```python
from build123d import *

# Parameters (mm, degrees)
SKETCH1_R               = 1.6
SKETCH1_R_2             = 1.15
SKETCH1_R_3             = 1.33
BASE_SHAPE_DEPTH        = 1.75
MILLING_FILLETS_R       = 1
SKETCH3_R               = 3
SCREW_HEAD_CUT_DEPTH    = 0.3
SCREW_HEAD_CHAMFER_SIZE = 1.4


with BuildPart() as part:
    # Sketch1 → Base shape (new body)
    with BuildSketch(Plane(origin=(0, 0, 0), x_dir=(1, 0, 0), z_dir=(0, 1, 0))):
        with BuildLine():
            Line((15.5, 39.2), (-15.5, 39.2))
            ThreePointArc((-15.5, 39.2), (-18.328427125, 38.028427125), (-19.5, 35.2))
            Line((-19.5, 35.2), (-19.5, -19.5))
            Line((-19.5, -19.5), (19.5, -19.5))
            Line((19.5, -19.5), (19.5, 35.2))
            ThreePointArc((19.5, 35.2), (18.328427125, 38.028427125), (15.5, 39.2))
        make_face()
        with Locations(Location((-15.25, -15.25, 0), (0, 0, 270))):
            Circle(SKETCH1_R, mode=Mode.SUBTRACT)
        with Locations(Location((15.25, -15.25, 0), (0, 0, 270))):
            Circle(SKETCH1_R, mode=Mode.SUBTRACT)
        with BuildLine():
            ThreePointArc((-17.7, 13.606832327), (-13.284874461, 13.049822367), (-13.341630288, 17.499583304))
            Line((-13.341630288, 17.499583304), (7.05, 17.499583304))
            Line((7.05, 17.499583304), (7.05, 17.05))
            ThreePointArc((7.05, 17.05), (8.336587223, 15.08098543), (10.656528722, 15.46853736))
            ThreePointArc((10.656528722, 15.46853736), (11.674639953, 15.673161101), (12.325380263, 14.863866097))
            ThreePointArc((12.325380263, 14.863866097), (14.578174541, 12.377518398), (17.7, 13.606832327))
            Line((17.7, 13.606832327), (17.7, -13.606832327))
            ThreePointArc((17.7, -13.606832327), (13.284874461, -13.049822367), (13.341630288, -17.499583304))
            Line((13.341630288, -17.499583304), (-13.341630288, -17.499583304))
            ThreePointArc((-13.341630288, -17.499583304), (-13.284874461, -13.049822367), (-17.7, -13.606832327))
            Line((-17.7, -13.606832327), (-17.7, 13.606832327))
        make_face(mode=Mode.SUBTRACT)
        with Locations(Location((-15.25, 15.25, 0), (0, 0, 270))):
            Circle(SKETCH1_R, mode=Mode.SUBTRACT)
        with Locations(Location((-15.25, 33.25, 0), (0, 0, 270))):
            Circle(SKETCH1_R, mode=Mode.SUBTRACT)
        with Locations(Location((9.2, 17.05, 0), (0, 0, 270))):
            Circle(SKETCH1_R_2, mode=Mode.SUBTRACT)
        with Locations(Location((15.25, 15.25, 0), (0, 0, 270))):
            Circle(SKETCH1_R, mode=Mode.SUBTRACT)
        with Locations(Location((3.5, 26.95, 0), (0, 0, 270))):
            Circle(SKETCH1_R_3, mode=Mode.SUBTRACT)
        with Locations(Location((15.25, 33.25, 0), (0, 0, 270))):
            Circle(SKETCH1_R, mode=Mode.SUBTRACT)
    extrude(amount=BASE_SHAPE_DEPTH)

    # Milling fillets
    milling_fillets_edges = [part.edges().sort_by_distance(p)[0] for p in [
        (-17.7, 0.875, 13.606832327),
        (-13.341630288, 0.875, 17.499583304),
        (13.341630288, 0.875, 17.499583304),
        (17.7, 0.875, 13.606832327),
        (17.7, 0.875, -13.606832327),
        (-13.341630288, 0.875, -17.499583304),
        (-17.7, 0.875, -13.606832327),
        (7.05, 0.875, -17.499583304),
    ]]
    fillet(milling_fillets_edges, radius=MILLING_FILLETS_R)

    # Sketch3 → Screw head cut (cut)
    with BuildSketch(Plane(origin=(0, 1.75, 0), x_dir=(1, 0, 0), z_dir=(0, 1, 0))):
        with Locations(Location((-15.25, 33.25, 0), (0, 0, 270))):
            Circle(SKETCH3_R)
        with Locations(Location((15.25, 33.25, 0), (0, 0, 270))):
            Circle(SKETCH3_R)
    extrude(amount=-SCREW_HEAD_CUT_DEPTH, mode=Mode.SUBTRACT)

    # Screw head chamfer
    screw_head_chamfer_edges = [part.edges().sort_by_distance(p)[0] for p in [
        (-15.25, 1.45, -34.85),
        (15.25, 1.45, -34.85),
    ]]
    chamfer(screw_head_chamfer_edges, length=SCREW_HEAD_CHAMFER_SIZE - 0.0001)  # a hair under: the kernel refuses the full size


solid = part.part
```
CAD build for the part. Positions are in the model's coordinates, mm. A direction names the side the tool comes from. Round coordinates to 2 decimals unless told otherwise and drop trailing zeros. Order: outer loops, then holes, each group sorted by start corner. A loop starts at its lowest first (then second) coordinate and runs counter-clockwise, first axis right, second up.
Item 1: Saw through at A-A on x = -1. Write the cut outline in (y, z), then the cut area to 3 significant figures.
Item 2: Saw through at C-C on z = -33.25. State how many separate pieces and enclosed holes the cut face has, then the cut area to 3 significant figures.
Item 3: Probe line 1 along X through (y, z) = (0.05, -33.25); line 2 along X through (y, z) = (1.55, -33.25); line 3 along X through (y, z) = (0.85, 15.25). List the from-to ranges inside material, lowest first.
Item 4: Saw through at B-B on z = -26.95. Write the cut outline in (x, y), then the cut area to 3 significant figures.
Item 5: Tool access for faces 5 (the face through (-12.322, 0.887, -17.073)), 6 (the face through (0, 1, -39.2)): list every direction of +Z, -Z, +X, -X, +Y, -Y with a clear straight run to the whole face (end or side of a thin tool).
Item 6: Mould opens along Z. For faces 1 (the face through (-12.322, 0.887, 17.073)), 2 (the face through (-18.297, 0.863, -38.059)), 3 (the face through (3.9, 0.86, -25.68)), 4 (the face through (-19.5, 1, -8)) say: pulls with the +Z half, pulls with the -Z half, needs draft (parallel to the pull), parting line crosses it, or undercut.
Item 7: Pin check, flat tips, straight feed: pin 1 (1.4 mm diameter, centred on x = 9.2, z = -17.05, fed in from +Y); pin 2 (1.8 mm diameter, centred on x = -16, z = -33.5, fed in from +Y); pin 3 (5 mm diameter, centred on x = 15.25, z = -33.25, fed in from +Y). Stop position of each tip, or through.
Reported:
1. outline: (0, -39.2) - (1.75, -39.2) - (1.75, -17.5) - (0, -17.5) - close; (0, 17.5) - (1.75, 17.5) - (1.75, 19.5) - (0, 19.5) - close
1. area: 41.5 mm2
2. separate pieces: 3
2. enclosed holes: 0
2. area: 51.5 mm2
3. line 1: x = -19.5 to -16.85, -13.65 to 13.65, 16.85 to 19.5
3. line 2: x = -19.5 to -18.25, -12.25 to 12.25, 18.25 to 19.5
3. line 3: x = -19.5 to -16.85, -13.65 to -12.3, 12.3 to 13.65, 16.85 to 19.5
4. outline: (-19.5, 0) - (2.17, 0) - (2.17, 1.75) - (-19.5, 1.75) - close; (4.83, 0) - (19.5, 0) - (19.5, 1.75) - (4.83, 1.75) - close
4. area: 63.6 mm2
5. face 5: +Y, -Y
5. face 6: -Z, +X, -X, +Y, -Y
6. face 1: undercut
6. face 2: pulls with the -Z half
6. face 3: undercut
6. face 4: needs draft
7. pin 1: passes through
7. pin 2: stops at y = 0.14
7. pin 3: stops at y = 0.95
